Here's how the part is built. I have some questions about the finished solid (model axes, mm). A direction names the side the tool comes from. Coordinates: 2 decimals unless noted, no trailing zeros. Write each loop counter-clockwise with the first axis right and the second up, starting at its lowest first coordinate (ties: lowest second). Pieces come first, ordered by that corner, then holes.
Item 1: If we section it at A-A (z = 18): Please give me the cut outline in (x, y).
Item 2: For faces 1 (the face through (59.074, 27.26, 17.596)), 2 (the face through (-56.65, 26.01, 19.57)), which set-ups out of +Z, -Z, +X, -X, +Y, -Y let a thin tool reach every point of the face, with its end or its side?
Item 3: If we section it at C-C (x = -36): Please give me the cut outline in (y, z), then the cut area to 3 significant figures.
Item 4: I'm going to push flat-ended pins straight in: pin 1 Ø0.6 at (x, y) = (-4, 25) entering from -Z; pin 2 Ø3 at (x, z) = (-56, -18.5) entering from +Y; pin 3 Ø24 at (x, z) = (12, -0.5) entering from -Y. Where does each tip first touch, or does it pass through?
Item 5: If we section it at D-D (z = -11.5): Please give me the cut outline in (x, y), then the cut area to 3 significant figures.
Item 6: If we section it at B-B (x = 56): Please give me the cut outline in (y, z), then the cut area to 3 significant figures.
Item 7: If I drill on line 1 (Z direction, x = 11.5, y = 25.35); line 2 (X direction, y = 25.1, z = 1); line 3 (X direction, y = 26.75, z = 20.5), over which ranges is the centre line in solid material (lowest first)?
Item 8: We'd pull the mould along Z, two halves only. Please class faces 3 (the face through (-1, 28, 0)), 4 (the face through (-52.926, 27.26, -18.404)): +Z half, -Z half, draft (parallel to the pull), parting line (faces both ways), or undercut.
from build123d import *

# Parameters (mm, degrees)
SKETCH1_W           = 126
SKETCH1_H           = 48
BOSS_EXTRUDE1_DEPTH = 2.5
CHAMFER1_SIZE       = 1
SKETCH2_W           = 119.4
SKETCH2_H           = 41.4
SKETCH2_W_2         = 116.2
SKETCH2_H_2         = 38.2
BOSS_EXTRUDE2_DEPTH = 1.2
SKETCH3_R           = 4.5
CUT_EXTRUDE1_DEPTH  = 1.5
SKETCH4_R           = 1.7
CUT_EXTRUDE2_DEPTH  = 68.518071655
SKETCH5_R           = 3.1
CUT_EXTRUDE3_DEPTH  = 1.5


with BuildPart() as part:
    # Sketch1 → Boss-Extrude1 (new body)
    with BuildSketch(Plane(origin=(0, 25.5, 0), x_dir=(1, 0, 0), z_dir=(0, 1, 0))):
        Rectangle(SKETCH1_W, SKETCH1_H)
    extrude(amount=BOSS_EXTRUDE1_DEPTH)

    # Chamfer1
    chamfer1_edges = [part.edges().sort_by_distance(p)[0] for p in [
        (63, 28, 0),
        (0, 28, -24),
        (-63, 28, 0),
        (0, 28, 24),
    ]]
    chamfer(chamfer1_edges, length=CHAMFER1_SIZE)

    # Sketch2 → Boss-Extrude2 (add)
    with BuildSketch(Plane(origin=(0, 25.5, 0), x_dir=(1, 0, 0), z_dir=(0, 1, 0))):
        Rectangle(SKETCH2_W, SKETCH2_H)
        Rectangle(SKETCH2_W_2, SKETCH2_H_2, mode=Mode.SUBTRACT)
    extrude(amount=-BOSS_EXTRUDE2_DEPTH)

    # Sketch3 → Cut-Extrude1 (cut)
    with BuildSketch(Plane(origin=(0, 25.5, 0), x_dir=(1, 0, 0), z_dir=(0, 1, 0))):
        with Locations((-56, 18)):
            Circle(SKETCH3_R)
        with Locations((-56, -18)):
            Circle(SKETCH3_R)
        with Locations((56, 18)):
            Circle(SKETCH3_R)
        with Locations((56, -18)):
            Circle(SKETCH3_R)
    extrude(amount=-CUT_EXTRUDE1_DEPTH, mode=Mode.SUBTRACT)

    # Sketch4 → Cut-Extrude2 (cut, through all)
    with BuildSketch(Plane(origin=(0, 28, 0), x_dir=(1, 0, 0), z_dir=(0, 1, 0))):
        with Locations(Location((-56, 18, 0), (0, 0, 270))):
            Circle(SKETCH4_R)
        with Locations(Location((-56, -18, 0), (0, 0, 270))):
            Circle(SKETCH4_R)
        with Locations(Location((56, 18, 0), (0, 0, 270))):
            Circle(SKETCH4_R)
        with Locations(Location((56, -18, 0), (0, 0, 270))):
            Circle(SKETCH4_R)
    extrude(amount=-CUT_EXTRUDE2_DEPTH, mode=Mode.SUBTRACT)

    # Sketch5 → Cut-Extrude3 (cut)
    with BuildSketch(Plane(origin=(0, 28, 0), x_dir=(1, 0, 0), z_dir=(0, 1, 0))):
        with Locations(Location((-56, 18, 0), (0, 0, 270))):
            Circle(SKETCH5_R)
        with Locations(Location((-56, -18, 0), (0, 0, 270))):
            Circle(SKETCH5_R)
        with Locations(Location((56, 18, 0), (0, 0, 270))):
            Circle(SKETCH5_R)
        with Locations(Location((56, -18, 0), (0, 0, 270))):
            Circle(SKETCH5_R)
    extrude(amount=-CUT_EXTRUDE3_DEPTH, mode=Mode.SUBTRACT)


solid = part.part
Answer list:
1. outline: (-63, 25.5) - (-57.7, 25.5) - (-57.7, 26.5) - (-59.1, 26.5) - (-59.1, 28) - (-62, 28) - (-63, 27) - close; (-54.3, 25.5) - (54.3, 25.5) - (54.3, 26.5) - (52.9, 26.5) - (52.9, 28) - (-52.9, 28) - (-52.9, 26.5) - (-54.3, 26.5) - close; (57.7, 25.5) - (63, 25.5) - (63, 27) - (62, 28) - (59.1, 28) - (59.1, 26.5) - (57.7, 26.5) - close
2. face 1: +Y
2. face 2: +Y, -Y
3. outline: (24.3, -20.7) - (25.5, -20.7) - (25.5, -24) - (27, -24) - (28, -23) - (28, 23) - (27, 24) - (25.5, 24) - (25.5, 20.7) - (24.3, 20.7) - (24.3, 19.1) - (25.5, 19.1) - (25.5, -19.1) - (24.3, -19.1) - close
3. area: 123 mm2
4. pin 1: stops at z = -20.7
4. pin 2: stops at y = 26.5
4. pin 3: stops at y = 25.5
5. outline: (-63, 25.5) - (-59.7, 25.5) - (-59.7, 24.3) - (-58.1, 24.3) - (-58.1, 25.5) - (58.1, 25.5) - (58.1, 24.3) - (59.7, 24.3) - (59.7, 25.5) - (63, 25.5) - (63, 27) - (62, 28) - (-62, 28) - (-63, 27) - close
5. area: 318 mm2
6. outline: (25.5, -24) - (27, -24) - (28, -23) - (28, -21.1) - (26.5, -21.1) - (26.5, -19.7) - (25.5, -19.7) - close; (25.5, -16.3) - (26.5, -16.3) - (26.5, -14.9) - (28, -14.9) - (28, 14.9) - (26.5, 14.9) - (26.5, 16.3) - (25.5, 16.3) - close; (25.5, 19.7) - (26.5, 19.7) - (26.5, 21.1) - (28, 21.1) - (28, 23) - (27, 24) - (25.5, 24) - close
6. area: 93.6 mm2
7. line 1: z = -20.7 to -19.1, 19.1 to 20.7
7. line 2: x = -59.7 to -58.1, 58.1 to 59.7
7. line 3: x = -63 to -57.83, -54.17 to 54.17, 57.83 to 63
8. face 3: draft
8. face 4: undercut
